from build123d import *

# Parameters (mm, degrees)
EXTRUDE_635_DEPTH      = 4.5
EXTRUDE_635_DEPTH_BACK = 4.5
SKETCH_1_R             = 3.2
SKETCH_3_R             = 3.65
CUT_EXTRUDE_1173_DEPTH = 3
SKETCH_5_R             = 3.75
EXTRUDE_1353_DEPTH     = 3
FILLET_3_R             = 1.5


with BuildPart() as part:
    # Sketch 1 → Extrude 635 (new, two sides: drawn at the far end of the back side and taken through both)
    with BuildSketch(Plane.XY.offset(-EXTRUDE_635_DEPTH_BACK)):
        Polygon((0, 10), (55, 10), (60, 15), (80, 15), (80, 0), (65, 0), (65, 2.5), (60, 2.5), (60, 0), (13, 0), (0, 0), align=None)
        with Locations((70, 7.5)):
            Circle(SKETCH_1_R, mode=Mode.SUBTRACT)
    extrude(amount=EXTRUDE_635_DEPTH + EXTRUDE_635_DEPTH_BACK)

    # Sketch 3 → Cut-Extrude 1173 (cut)
    with BuildSketch(Plane.XY.offset(4.5)):
        with Locations((70, 7.5)):
            Circle(SKETCH_3_R)
    cut_extrude_1173 = extrude(amount=-CUT_EXTRUDE_1173_DEPTH, mode=Mode.SUBTRACT)

    # Mirror 1: Cut-Extrude 1173 across plane
    add(cut_extrude_1173.mirror(Plane.XY), mode=Mode.SUBTRACT)

    # Sketch 5 → Extrude 1353 (add)
    with BuildSketch(Plane(origin=(0, 10, 0), x_dir=(1, 0, 0), z_dir=(0, 1, 0))):
        with Locations(Location((20, 0, 0), (0, 0, 270))):
            Circle(SKETCH_5_R)
    extrude(amount=EXTRUDE_1353_DEPTH)

    # Fillet 3
    fillet_3_edges = [part.edges().sort_by_distance(p)[0] for p in [
        (20, 13, -3.75),
    ]]
    fillet(fillet_3_edges, radius=FILLET_3_R)


solid = part.part
CAD build for the part. Positions are in the model's coordinates, mm. A direction names the side the tool comes from. Round coordinates to 2 decimals unless told otherwise and drop trailing zeros. Loops run counter-clockwise (first coordinate to the right, second up) from the corner with the lowest first, then second, coordinate; pieces in that order, holes last.
(1) Cut at B-B (x = 70). Give the cut face in (y, z), plus the area to 3 significant figures.
(2) Cut at C-C (z = 0). Give the cut face in (x, y), plus the area to 3 significant figures.
(3) Cut at D-D (x = 20). Give the cut face in (y, z).
(4) Wall check: line 1 along Y through (x, z) = (70, 2.55); line 2 along Y through (x, z) = (70, 0.15); line 3 along Y through (x, z) = (27.5, -0.5). Give the ranges that are in metal, low to high.
(5) Drop flat-ended pins along their axis: pin 1 (2 mm diameter, centred on x = 69, y = 6, fed in from +Z); pin 2 (2 mm diameter, centred on x = 21, z = 0, fed in from +Y); pin 3 (1.5 mm diameter, centred on x = 62, z = -1.5, fed in from -Y). Give the stop position or say it passes through.
(6) Cut at A-A (y = 7.5). Give the cut face in (x, z), plus the area to 3 significant figures.
(7) Which spindle directions (+Z, -Z, +X, -X, +Y, -Y) get a long thin tool onto all of the face, cutting with end or side? Do faces 1 (the flat face through (57, 12, 0)), 2 (the cylindrical face through (73.48, 8.6, -3.02)), 3 (the cylindrical face through (73.48, 8.6, 3.02)), 4 (the flat face through (63, 2.5, 0)). Say none if no direction does.
(8) Two-plate mould, pull along X, no slides. Class faces 5 (the cylindrical face through (16.34, 10.74, -0.81)), 6 (the flat face through (20, 13, 0)), 7 (the flat face through (0, 5, 0)): +X half, -X half, draft (parallel to the pull), parting line (faces both ways), or undercut.
Findings below:
1. outline: (0, -4.5) - (3.85, -4.5) - (3.85, -1.5) - (4.3, -1.5) - (4.3, 1.5) - (3.85, 1.5) - (3.85, 4.5) - (0, 4.5) - close; (10.7, -1.5) - (11.15, -1.5) - (11.15, -4.5) - (15, -4.5) - (15, 4.5) - (11.15, 4.5) - (11.15, 1.5) - (10.7, 1.5) - close
1. area: 72.0 mm2
2. outline: (0, 0) - (60, 0) - (60, 2.5) - (65, 2.5) - (65, 0) - (80, 0) - (80, 15) - (60, 15) - (55, 10) - (23.75, 10) - (23.75, 11.5) arc R1.5 ccw to (22.25, 13) - (17.75, 13) arc R1.5 ccw to (16.25, 11.5) - (16.25, 10) - (0, 10) - close; hole circle Ø6.4 at (70, 7.5)
2. area: 889 mm2
3. outline: (0, -4.5) - (10, -4.5) - (10, -3.75) - (11.5, -3.75) arc R1.5 ccw to (13, -2.25) - (13, 2.25) arc R1.5 ccw to (11.5, 3.75) - (10, 3.75) - (10, 4.5) - (0, 4.5) - close
4. line 1: y = 0 to 3.85, 11.15 to 15
4. line 2: y = 0 to 4.3, 10.7 to 15
4. line 3: y = 0 to 10
5. pin 1: passes through
5. pin 2: stops at y = 13
5. pin 3: stops at y = 2.5
6. outline: (0, -4.5) - (66.35, -4.5) - (66.35, -1.5) - (66.8, -1.5) - (66.8, 1.5) - (66.35, 1.5) - (66.35, 4.5) - (0, 4.5) - close; (73.2, -1.5) - (73.65, -1.5) - (73.65, -4.5) - (80, -4.5) - (80, 4.5) - (73.65, 4.5) - (73.65, 1.5) - (73.2, 1.5) - close
6. area: 657 mm2
7. face 1: +Z, -Z, +Y
7. face 2: -Z
7. face 3: +Z
7. face 4: +Z, -Z, -Y
8. face 5: undercut
8. face 6: draft
8. face 7: -X half
